Geometry check sheet. Reference: the model listing, model coordinates, mm. Face numbers are marked on the shaded views. A direction names the side the tool comes from. Give positions to 0.01 mm unless a question says otherwise; leave off trailing zeros. Write each loop counter-clockwise with the first axis right and the second up, starting at its lowest first coordinate (ties: lowest second). Pieces come first, ordered by that corner, then holes. Notation, with made-up numbers: (30.25, 29.25) - (54.25, 29.25) arc R17 cw to (54.25, 56.25) - close; hole circle Ø1 at (11.5, 14.25). An arc over 180 degrees is marked (long way). Use a Markdown table: item, result.
```python
from build123d import *

# Parameters (mm, degrees)
ESQUISSE1_W             = 36
ESQUISSE1_H             = 36
ESQUISSE1_R             = 1.1
ESQUISSE1_R_2           = 4.4
ESQUISSE1_R_3           = 1.6
BOSS_EXTRU_1_DEPTH      = 3
ESQUISSE2_R             = 3
BOSS_EXTRU_2_DEPTH      = 1.6
ESQUISSE3_R             = 1.5
ENL_V_MAT_EXTRU_1_DEPTH = 26.868127107
CONG_1_R                = 2
BOSS_EXTRU_3_DEPTH      = 6
BOSS_EXTRU_3_DEPTH_BACK = 3
ESQUISSE4_R             = 2.2
CONG_2_R                = 4
CONG_3_R                = 4


with BuildPart() as part:
    # Esquisse1 → Boss.-Extru.1 (new body)
    with BuildSketch(Plane.XY):
        Rectangle(ESQUISSE1_W, ESQUISSE1_H)
        with Locations((-4.242640687, 4.242640687)):
            Circle(ESQUISSE1_R, mode=Mode.SUBTRACT)
        with Locations((4.242640687, 4.242640687)):
            Circle(ESQUISSE1_R, mode=Mode.SUBTRACT)
        with Locations((4.242640687, -4.242640687)):
            Circle(ESQUISSE1_R, mode=Mode.SUBTRACT)
        with Locations((-4.242640687, -4.242640687)):
            Circle(ESQUISSE1_R, mode=Mode.SUBTRACT)
        Circle(ESQUISSE1_R_2, mode=Mode.SUBTRACT)
        with Locations((-15, 15)):
            Circle(ESQUISSE1_R_3, mode=Mode.SUBTRACT)
        with Locations(Location((15, 15, 0), (0, 0, 180))):
            Circle(ESQUISSE1_R_3, mode=Mode.SUBTRACT)
        with Locations((15, -15)):
            Circle(ESQUISSE1_R_3, mode=Mode.SUBTRACT)
        with Locations(Location((-15, -15, 0), (0, 0, 180))):
            Circle(ESQUISSE1_R_3, mode=Mode.SUBTRACT)
    extrude(amount=BOSS_EXTRU_1_DEPTH)

    # Esquisse2 → Boss.-Extru.2 (add)
    with BuildSketch(Plane.XY.offset(3)):
        with Locations((-8, 8)):
            Circle(ESQUISSE2_R)
        with Locations((8, 8)):
            Circle(ESQUISSE2_R)
        with Locations((8, -8)):
            Circle(ESQUISSE2_R)
        with Locations((-8, -8)):
            Circle(ESQUISSE2_R)
    extrude(amount=BOSS_EXTRU_2_DEPTH)

    # Esquisse3 → Enlèv. mat.-Extru.1 (cut, through all)
    with BuildSketch(Plane.XY.offset(4.6)):
        with Locations((-8, 8)):
            Circle(ESQUISSE3_R)
        with Locations(Location((8, 8, 0), (0, 0, 180))):
            Circle(ESQUISSE3_R)
        with Locations((8, -8)):
            Circle(ESQUISSE3_R)
        with Locations(Location((-8, -8, 0), (0, 0, 180))):
            Circle(ESQUISSE3_R)
    extrude(amount=-ENL_V_MAT_EXTRU_1_DEPTH, mode=Mode.SUBTRACT)

    # Congé1
    cong_1_edges = [part.edges().sort_by_distance(p)[0] for p in [
        (-18, 18, 1.5),
        (18, 18, 1.5),
        (18, -18, 1.5),
        (-18, -18, 1.5),
    ]]
    fillet(cong_1_edges, radius=CONG_1_R)

    # Esquisse4 → Boss.-Extru.3 (add, two sides: drawn at the far end of the back side and taken through both)
    # profile 1 of 4: a face of its own
    with BuildSketch(Plane.XY.offset(3).offset(-BOSS_EXTRU_3_DEPTH_BACK)):
        with BuildLine():
            Line((-6, 30), (-6, 18))
            Line((-6, 18), (6, 18))
            Line((6, 18), (6, 30))
            ThreePointArc((6, 30), (0, 36), (-6, 30))
        make_face()
        with Locations((0, 30)):
            Circle(ESQUISSE4_R, mode=Mode.SUBTRACT)
    # profile 2 of 4: a face of its own
    with BuildSketch(Plane.XY.offset(3).offset(-BOSS_EXTRU_3_DEPTH_BACK)):
        with BuildLine():
            Line((30, 6), (18, 6))
            Line((18, 6), (18, -6))
            Line((18, -6), (30, -6))
            ThreePointArc((30, -6), (36, 0), (30, 6))
        make_face()
        with Locations((30, 0)):
            Circle(ESQUISSE4_R, mode=Mode.SUBTRACT)
    # profile 3 of 4: a face of its own
    with BuildSketch(Plane.XY.offset(3).offset(-BOSS_EXTRU_3_DEPTH_BACK)):
        with BuildLine():
            Line((6, -30), (6, -18))
            Line((6, -18), (-6, -18))
            Line((-6, -18), (-6, -30))
            ThreePointArc((-6, -30), (0, -36), (6, -30))
        make_face()
        with Locations((0, -30)):
            Circle(ESQUISSE4_R, mode=Mode.SUBTRACT)
    # profile 4 of 4: a face of its own
    with BuildSketch(Plane.XY.offset(3).offset(-BOSS_EXTRU_3_DEPTH_BACK)):
        with BuildLine():
            Line((-30, -6), (-18, -6))
            Line((-18, -6), (-18, 6))
            Line((-18, 6), (-30, 6))
            ThreePointArc((-30, 6), (-36, 0), (-30, -6))
        make_face()
        with Locations((-30, 0)):
            Circle(ESQUISSE4_R, mode=Mode.SUBTRACT)
    extrude(amount=BOSS_EXTRU_3_DEPTH + BOSS_EXTRU_3_DEPTH_BACK)

    # Congé2
    cong_2_edges = [part.edges().sort_by_distance(p)[0] for p in [
        (6, 18, 6),
        (-6, 18, 6),
        (18, -6, 6),
        (18, 6, 6),
        (-6, -18, 6),
        (6, -18, 6),
        (-18, 6, 6),
        (-18, -6, 6),
    ]]
    fillet(cong_2_edges, radius=CONG_2_R)

    # Congé3
    cong_3_edges = [part.edges().sort_by_distance(p)[0] for p in [
        (18, -6, 1.5),
        (18, 6, 1.5),
        (6, 18, 1.5),
        (-6, 18, 1.5),
        (-18, 6, 1.5),
        (-18, -6, 1.5),
        (-6, -18, 1.5),
        (6, -18, 1.5),
    ]]
    fillet(cong_3_edges, radius=CONG_3_R)


solid = part.part
```
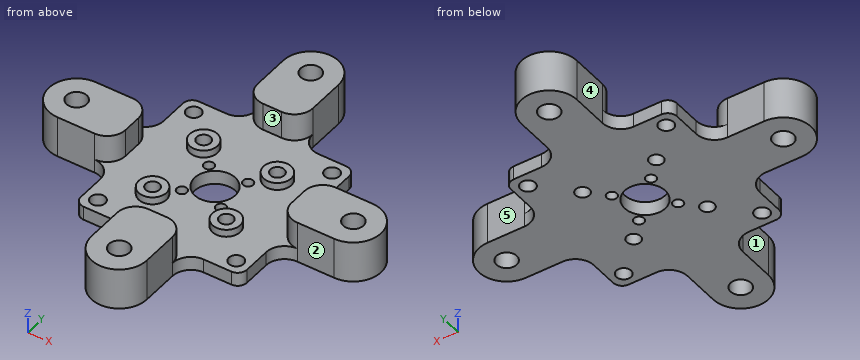
1) Section check D-D on x = 8. Record the boundary of the cut face in (y, z), then the cut area to 3 significant figures.
Working result:
| item | result |
|---|---|
| outline | (-18.54, 0) - (-9.5, 0) - (-9.5, 4.6) - (-11, 4.6) - (-11, 3) - (-18.54, 3) - close; (-6.5, 0) - (6.5, 0) - (6.5, 4.6) - (5, 4.6) - (5, 3) - (-5, 3) - (-5, 4.6) - (-6.5, 4.6) - close; (9.5, 0) - (18.54, 0) - (18.54, 3) - (11, 3) - (11, 4.6) - (9.5, 4.6) - close |
| area | 103 mm² |
2) Section check B-B on x = -15. Record the boundary of the cut face in (y, z), then the cut area to 3 significant figures.
Working result:
| item | result |
|---|---|
| outline | (-18, 0) - (-16.6, 0) - (-16.6, 3) - (-18, 3) - close; (-13.4, 0) - (13.4, 0) - (13.4, 3) - (-13.4, 3) - close; (16.6, 0) - (18, 0) - (18, 3) - (16.6, 3) - close |
| area | 88.8 mm² |
3) Depth check by flat-ended pin: P1, Ø4, axis at x = 0, y = -30, coming from the +Z side; P2, Ø7, axis at x = -30, y = 0, coming from the +Z side; P3, Ø2.5, axis at y = -27, z = 6.5, coming from the +X side; P4, Ø4, axis at y = 25, z = 4, coming from the -X side. Enter the tip coordinate at first touch or a pass-through.
Working result:
| item | result |
|---|---|
| P1 | passes through |
| P2 | stops at z = 9 |
| P3 | stops at x = 6 |
| P4 | stops at x = -6 |
4) Section check A-A on y = 0. Record the boundary of the cut face in (x, z).
Working result:
| item | result |
|---|---|
| outline | (-36, 0) - (-32.2, 0) - (-32.2, 9) - (-36, 9) - close; (-27.8, 0) - (-4.4, 0) - (-4.4, 3) - (-18, 3) - (-18, 9) - (-27.8, 9) - close; (4.4, 0) - (27.8, 0) - (27.8, 9) - (18, 9) - (18, 3) - (4.4, 3) - close; (32.2, 0) - (36, 0) - (36, 9) - (32.2, 9) - close |
5) Material ranges on L1, parallel to Y at x = -30, z = 2; L2, parallel to Y at x = 24, z = 2.25; L3, parallel to Z at x = -15.5, y = -13, recorded low to high. Write a range as from..to.
Working result:
| item | result |
|---|---|
| L1 | y = -6..-2.2, 2.2..6 |
| L2 | y = -6..6 |
| L3 | z = 0..3 |
6) Set-up check for the marked faces 1, 2, 3, 4 and 5: record each of +Z, -Z, +X, -X, +Y, -Y from which the full face is reachable in a straight line by a thin tool's end or side.
Working result:
| item | result |
|---|---|
| face 1 | +Z, -Z, -X, -Y |
| face 2 | +Z, -Z, +X, -Y |
| face 3 | +Z, +X, -X |
| face 4 | +Z, -Z, -X, +Y |
| face 5 | +Z, -Z, +X, +Y |
